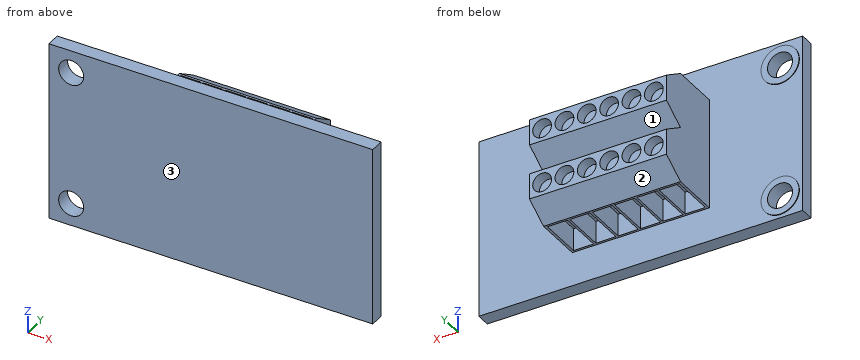
```python
from build123d import *

# Parameters (mm, degrees)
SKETCH1_W           = 36.83
SKETCH1_H           = 20.32
BOSS_EXTRUDE1_DEPTH = 1.6002
SKETCH5_R           = 1.4224
CUT_EXTRUDE3_DEPTH  = 22.092616363
BOSS_EXTRUDE2_DEPTH = 7.7851
BOSS_EXTRUDE3_DEPTH = 7.7851
SKETCH11_W          = 2.286
SKETCH11_H          = 4.953
CUT_EXTRUDE5_DEPTH  = 2.54
SKETCH12_W          = 2.286
SKETCH12_H          = 4.953
CUT_EXTRUDE6_DEPTH  = 2.54
SKETCH13_R          = 1.0668
CUT_EXTRUDE7_DEPTH  = 1.27
SKETCH17_R          = 1.0668
CUT_EXTRUDE9_DEPTH  = 1.27
SKETCH21_R          = 2.159
SKETCH21_R_2        = 1.4224
BOSS_EXTRUDE5_DEPTH = 0.0762


with BuildPart() as part:
    # Sketch1 → Boss-Extrude1 (new body)
    with BuildSketch(Plane(origin=(0, 0, 0), x_dir=(1, 0, 0), z_dir=(0, 1, 0))):
        Rectangle(SKETCH1_W, SKETCH1_H)
    extrude(amount=BOSS_EXTRUDE1_DEPTH)

    # Sketch5 → Cut-Extrude3 (cut, through all)
    with BuildSketch(Plane(origin=(0, 0, 0), x_dir=(1, 0, 0), z_dir=(0, 1, 0))):
        with Locations(Location((-15.875, 7.62, 0), (0, 0, 270))):
            Circle(SKETCH5_R)
        with Locations(Location((-15.875, -7.62, 0), (0, 0, 270))):
            Circle(SKETCH5_R)
    extrude(amount=CUT_EXTRUDE3_DEPTH, mode=Mode.SUBTRACT)

    # Sketch8 → Boss-Extrude2 (add, symmetric)
    with BuildSketch(Plane(origin=(0, 0, 0), x_dir=(0, 0, -1), z_dir=(1, 0, 0))):
        Polygon((0, 1.6002), (6.2992, 1.6002), (6.2992, 7.0612), (4.6101, 9.742765812), (1.6891, 9.742765812), (0, 7.0612), align=None)
    extrude(amount=BOSS_EXTRUDE2_DEPTH, both=True)

    # Sketch10 → Boss-Extrude3 (add, symmetric)
    with BuildSketch(Plane(origin=(0, 0, 0), x_dir=(0, 0, -1), z_dir=(1, 0, 0))):
        Polygon((-6.2992, 1.6002), (0, 1.6002), (0, 7.0612), (-1.6891, 9.742765812), (-4.6101, 9.742765812), (-6.2992, 7.0612), align=None)
    extrude(amount=BOSS_EXTRUDE3_DEPTH, both=True)

    # Sketch11 → Cut-Extrude5 (cut)
    with BuildSketch(Plane.XY.offset(6.2992)):
        with Locations((-1.27, 4.3307)):
            Rectangle(SKETCH11_W, SKETCH11_H)
        with Locations((-3.81, 4.3307)):
            Rectangle(SKETCH11_W, SKETCH11_H)
        with Locations((-6.35, 4.3307)):
            Rectangle(SKETCH11_W, SKETCH11_H)
        with Locations((1.27, 4.3307)):
            Rectangle(SKETCH11_W, SKETCH11_H)
        with Locations((3.81, 4.3307)):
            Rectangle(SKETCH11_W, SKETCH11_H)
        with Locations((6.35, 4.3307)):
            Rectangle(SKETCH11_W, SKETCH11_H)
    extrude(amount=-CUT_EXTRUDE5_DEPTH, mode=Mode.SUBTRACT)

    # Sketch12 → Cut-Extrude6 (cut)
    with BuildSketch(Plane(origin=(0, 0, -6.2992), x_dir=(-1, 0, 0), z_dir=(0, 0, -1))):
        with Locations((-1.27, 4.3307)):
            Rectangle(SKETCH12_W, SKETCH12_H)
        with Locations((-3.81, 4.3307)):
            Rectangle(SKETCH12_W, SKETCH12_H)
        with Locations((-6.35, 4.3307)):
            Rectangle(SKETCH12_W, SKETCH12_H)
        with Locations((1.27, 4.3307)):
            Rectangle(SKETCH12_W, SKETCH12_H)
        with Locations((3.81, 4.3307)):
            Rectangle(SKETCH12_W, SKETCH12_H)
        with Locations((6.35, 4.3307)):
            Rectangle(SKETCH12_W, SKETCH12_H)
    extrude(amount=-CUT_EXTRUDE6_DEPTH, mode=Mode.SUBTRACT)

    # Sketch13 → Cut-Extrude7 (cut)
    with BuildSketch(Plane(origin=(0, 9.742765812, 0), x_dir=(1, 0, 0), z_dir=(0, 1, 0))):
        with Locations(Location((-1.27, -3.1496, 0), (0, 0, 270))):
            Circle(SKETCH13_R)
        with Locations(Location((-3.81, -3.1496, 0), (0, 0, 270))):
            Circle(SKETCH13_R)
        with Locations(Location((-6.35, -3.1496, 0), (0, 0, 270))):
            Circle(SKETCH13_R)
        with Locations(Location((1.27, -3.1496, 0), (0, 0, 270))):
            Circle(SKETCH13_R)
        with Locations(Location((3.81, -3.1496, 0), (0, 0, 270))):
            Circle(SKETCH13_R)
        with Locations(Location((6.35, -3.1496, 0), (0, 0, 270))):
            Circle(SKETCH13_R)
    extrude(amount=-CUT_EXTRUDE7_DEPTH, mode=Mode.SUBTRACT)

    # Sketch17 → Cut-Extrude9 (cut)
    with BuildSketch(Plane(origin=(0, 9.742765812, 0), x_dir=(1, 0, 0), z_dir=(0, 1, 0))):
        with Locations(Location((-1.27, 3.1496, 0), (0, 0, 270))):
            Circle(SKETCH17_R)
        with Locations(Location((-3.81, 3.1496, 0), (0, 0, 270))):
            Circle(SKETCH17_R)
        with Locations(Location((-6.35, 3.1496, 0), (0, 0, 270))):
            Circle(SKETCH17_R)
        with Locations(Location((1.27, 3.1496, 0), (0, 0, 270))):
            Circle(SKETCH17_R)
        with Locations(Location((3.81, 3.1496, 0), (0, 0, 270))):
            Circle(SKETCH17_R)
        with Locations(Location((6.35, 3.1496, 0), (0, 0, 270))):
            Circle(SKETCH17_R)
    extrude(amount=-CUT_EXTRUDE9_DEPTH, mode=Mode.SUBTRACT)

    # Sketch21 → Boss-Extrude5 (add)
    # profile 1 of 2: a face of its own
    with BuildSketch(Plane(origin=(0, 1.6002, 0), x_dir=(1, 0, 0), z_dir=(0, 1, 0))):
        with Locations(Location((-15.875, -7.62, 0), (0, 0, 270))):
            Circle(SKETCH21_R)
        with Locations(Location((-15.875, -7.62, 0), (0, 0, 270))):
            Circle(SKETCH21_R_2, mode=Mode.SUBTRACT)
    # profile 2 of 2: a face of its own
    with BuildSketch(Plane(origin=(0, 1.6002, 0), x_dir=(1, 0, 0), z_dir=(0, 1, 0))):
        with Locations(Location((-15.875, 7.62, 0), (0, 0, 270))):
            Circle(SKETCH21_R)
        with Locations(Location((-15.875, 7.62, 0), (0, 0, 270))):
            Circle(SKETCH21_R_2, mode=Mode.SUBTRACT)
    extrude(amount=BOSS_EXTRUDE5_DEPTH)


solid = part.part
```
Can you work these out from the model? Positions are in its coordinate system, mm. Face numbers are marked on the shaded views. Give positions to 0.01 mm unless a question says otherwise; leave off trailing zeros. Write each loop counter-clockwise with the first axis right and the second up, starting at its lowest first coordinate (ties: lowest second). Pieces come first, ordered by that corner, then holes. Notation, with made-up numbers: (21.5, 14) -> (64.5, 14) arc R25 ccw to (64.5, 31) -> close; hole circle Ø3 at (69.25, -20.75). An arc over 180 degrees is marked (long way). Write item = value, one per line.
(1) Suppose I cut it at A-A on z = -7.62. Write out the boundary of the cut face in (x, y) (3 decimals), then the cut area to 3 significant figures.
Worked out:
outline = (-18.415, 0) -> (-17.297, 0) -> (-17.297, 1.676) -> (-18.034, 1.676) -> (-18.034, 1.6) -> (-18.415, 1.6) -> close; (-14.453, 0) -> (18.415, 0) -> (18.415, 1.6) -> (-13.716, 1.6) -> (-13.716, 1.676) -> (-14.453, 1.676) -> close
area = 54.5 mm^2
(2) I need wall thicknesses on probe 1 along Z at (x, y) = (4, 2.25); probe 2 along Y at (x, z) = (3, -4); probe 3 along X at (y, z) = (4.5, -0.5). Which ranges of each line are inside material? Lowest first, please. Write a range as from..to.
Worked out:
probe_1 = -3.76..3.76
probe_2 = 0..1.85, 6.81..9.74
probe_3 = -7.79..7.79
(3) Suppose I cut it at C-C on y = 1. Write out the boundary of the cut face in (x, z) (3 decimals).
Worked out:
outline = (-18.415, -10.16) -> (18.415, -10.16) -> (18.415, 10.16) -> (-18.415, 10.16) -> close; hole circle Ø2.845 at (-15.875, -7.62); hole circle Ø2.845 at (-15.875, 7.62)
(4) I'm going to push flat-ended pins straight in: P1, Ø5, axis at y = 5.5, z = 0, coming from the +X side; P2, Ø0.7, axis at x = -6.5, z = 4.5, coming from the -Y side; P3, Ø2.5, axis at x = 6, y = 4.5, coming from the +Z side; P4, Ø1.1, axis at x = 6.5, z = 5.5, coming from the +Y side. Where does each tip first touch, or does it pass through?
Worked out:
P1 = 7.79
P2 = 0
P3 = 6.3
P4 = 9.2
(5) Thinking about a two-plate mould opening in Z: for the marked faces 1, 2 and 3, which applies, released by +Z, released by -Z, zero draft, split by the parting line, or undercut?
Worked out:
face_1 = undercut
face_2 = released by -Z
face_3 = zero draft
